Geometry check sheet. Reference: the model listing, model coordinates, mm. A direction names the side the tool comes from. Round coordinates to 2 decimals unless told otherwise and drop trailing zeros. Order: outer loops, then holes, each group sorted by start corner. A loop starts at its lowest first (then second) coordinate and runs counter-clockwise, first axis right, second up. Notation, with made-up numbers: (5, 57.5) - (18, 57.5) arc R13 ccw to (18, 73.5) - close; hole circle Ø4 at (19.5, -30). An arc over 180 degrees is marked (long way). Use a Markdown table: item, result. Add a question column.
(1) Access from +Z, -Z, +X, -X, +Y, -Y to the whole of each face (thin tool, end or side, straight path). Record for faces 1 (the face through (0.5, 0, 3.7)), 2 (the face through (-1, 1, 4)).
(2) Section check B-B on x = 0.6. Record the boundary of the cut face in (y, z), then the cut area to 3 significant figures.
(3) Thickness scan on line 1 along Y through (x, z) = (0.5, 3.5); line 2 along X through (y, z) = (0.5, 5.75); line 3 along Y through (x, z) = (0.4, 1.25). Record the ranges inside material, lowest first. Write a range as [from, to].
(4) Mould release check, pull along Y, two halves, no side actions. Record for faces 3 (the face through (0, 1, 4)), 4 (the face through (-0.01, -0.24, 7.78)), 5 (the face through (1, -0.2, 3.5)), 6 (the face through (0.5, 2.6, 3.8)): released by +Y, released by -Y, zero draft, split by the parting line, or undercut.
(5) Section check C-C on y = 0.8. Record the boundary of the cut face in (x, z).
(6) Gauge pin test, flat end, axial feed: P1, Ø0.8, axis at y = 1.5, z = 2, coming from the +X side. Record the tip position at first contact, or that the pin passes through.
(7) Section check A-A on z = 5. Record the boundary of the cut face in (x, y).
(8) Section check D-D on x = -0.3. Record the boundary of the cut face in (y, z).
Autodesk Inventor part; units mm, degrees
ref_plane "YZ Plane" through (0, 0, 0) normal (1, 0, 0) x (0, 1, 0)
ref_plane "XZ Plane" through (0, 0, 0) normal (0, 1, 0) x (-1, 0, 0)
ref_plane "XY Plane" through (0, 0, 0) normal (0, 0, 1) x (1, 0, 0)
sketch "Skizze2" plane through (0, 0, 0) normal (1, 0, 0) x (0, 1, 0)
  arc A0 (0.4, 7.55) -> (0, 7.15) centre (0.4, 7.15) ccw
  line L0 (0.4, 7.55) -> (0.9477, 7.55)
  arc A1 (1.6402, 7.2714) -> (0.9477, 7.55) centre (0.9477, 6.55) ccw
  line L1 (1.6402, 7.2714) -> (2.2925, 6.6452)
  arc A2 (2.6, 5.9238) -> (2.2925, 6.6452) centre (1.6, 5.9238) ccw
  line L2 (2.6, 5.9238) -> (2.6, 1.6262)
  arc A3 (2.2925, 0.9048) -> (2.6, 1.6262) centre (1.6, 1.6262) ccw
  line L3 (2.2925, 0.9048) -> (1.6402, 0.2786)
  arc A4 (0.9477, 0) -> (1.6402, 0.2786) centre (0.9477, 1) ccw
  line L4 (0.9477, 0) -> (0.4, 0)
  arc A5 (0, 0.4) -> (0.4, 0) centre (0.4, 0.4) ccw
  line L5 (0, 0.4) -> (0, 7.15)
  line L6 (0.9477, 8.05) -> (0.4, 8.05)
  arc A6 (0.4, 8.05) -> (-0.5, 7.15) centre (0.4, 7.15) ccw
  line L7 (-0.5, 7.15) -> (-0.5, 0.4)
  arc A7 (-0.5, 0.4) -> (0.4, -0.5) centre (0.4, 0.4) ccw
  line L8 (0.4, -0.5) -> (0.9477, -0.5)
  arc A8 (0.9477, -0.5) -> (1.9865, -0.0821) centre (0.9477, 1) ccw
  line L9 (1.9865, -0.0821) -> (2.6388, 0.5441)
  arc A9 (2.6388, 0.5441) -> (3.1, 1.6262) centre (1.6, 1.6262) ccw
  line L10 (3.1, 1.6262) -> (3.1, 5.9238)
  arc A10 (3.1, 5.9238) -> (2.6388, 7.0059) centre (1.6, 5.9238) ccw
  line L11 (2.6388, 7.0059) -> (1.9865, 7.6321)
  arc A11 (1.9865, 7.6321) -> (0.9477, 8.05) centre (0.9477, 6.55) ccw
  point P0 (0, 0)
  dimension "d0" = 0.5
extrude "Extrusion1" add sketch "Skizze2" along normal blind 1
extrude "Extrusion2" add sketch "Skizze2" against normal blind 1 contours L0 A1 L1 A2 L2 A3 L3 A4 L4 A5 L5 A0 | A11 L11 A10 L10 A9 L9 A8 L8 A7 L7 A6 L6
properties part number "Power_Cap" material "PA 6.6"
Check sheet entries:
| question | item | result |
|---|---|---|
| 1 | face 1 | +X |
| 1 | face 2 | +Z, -Z, -X, +Y, -Y |
| 2 | outline | (-0.5, 0.4) arc R0.9 ccw to (0.4, -0.5) - (0.95, -0.5) arc R1.5 ccw to (1.99, -0.08) - (2.64, 0.54) arc R1.5 ccw to (3.1, 1.63) - (3.1, 5.92) arc R1.5 ccw to (2.64, 7.01) - (1.99, 7.63) arc R1.5 ccw to (0.95, 8.05) - (0.4, 8.05) arc R0.9 ccw to (-0.5, 7.15) - close; hole (0, 0.4) arc R0.4 ccw to (0.4, 0) - (0.95, 0) arc R1 ccw to (1.64, 0.28) - (2.29, 0.9) arc R1 ccw to (2.6, 1.63) - (2.6, 5.92) arc R1 ccw to (2.29, 6.65) - (1.64, 7.27) arc R1 ccw to (0.95, 7.55) - (0.4, 7.55) arc R0.4 ccw to (0, 7.15) - close |
| 2 | area | 9.96 mm2 |
| 3 | line 1 | y = [-0.5, 0], [2.6, 3.1] |
| 3 | line 2 | x = [-1, 0] |
| 3 | line 3 | y = [-0.5, 0], [2.53, 3.05] |
| 4 | face 3 | undercut |
| 4 | face 4 | released by -Y |
| 4 | face 5 | zero draft |
| 4 | face 6 | undercut |
| 5 | outline | (-1, -0.5) - (1, -0.5) - (1, 0) - (0, 0) - (0, 7.55) - (1, 7.55) - (1, 8.05) - (-1, 8.05) - close |
| 6 | P1 | stops at x = 0 |
| 7 | outline | (-1, -0.5) - (1, -0.5) - (1, 0) - (0, 0) - (0, 2.6) - (1, 2.6) - (1, 3.1) - (-1, 3.1) - close |
| 8 | outline | (-0.5, 0.4) arc R0.9 ccw to (0.4, -0.5) - (0.95, -0.5) arc R1.5 ccw to (1.99, -0.08) - (2.64, 0.54) arc R1.5 ccw to (3.1, 1.63) - (3.1, 5.92) arc R1.5 ccw to (2.64, 7.01) - (1.99, 7.63) arc R1.5 ccw to (0.95, 8.05) - (0.4, 8.05) arc R0.9 ccw to (-0.5, 7.15) - close |
